```python
from build123d import *

# Parameters (mm, degrees)
F0_R     = 12.7
F2_DEPTH = 362.63707
F3_D     = 19.05


with BuildPart() as f2:
    # F0 (on Right) → F2 (new body)
    with BuildSketch(Plane.YZ):
        Circle(F0_R)
    extrude(amount=F2_DEPTH)

    # F3 (through all)
    with Locations(Plane(origin=(0, 0, 0), x_dir=(0, 1, 0), z_dir=(-1, 0, 0))):
        with Locations((0, 0)):
            Hole(F3_D / 2)

    # F4: F2 across plane


with BuildPart() as f2_1:
    add(f2.part)
    add(f2.part.mirror(Plane.YZ))


solid = f2_1.part
```
Design review of the part built by this model. Coordinates are the model's own, in mm. Round coordinates to 2 decimals unless told otherwise and drop trailing zeros. Order: outer loops, then holes, each group sorted by start corner. A loop starts at its lowest first (then second) coordinate and runs counter-clockwise, first axis right, second up. Notation, with made-up numbers: M 33,-29 L 60,-29 A6 cw 60,-23 Z; hole C 39.5,30 d9. An arc over 180 degrees is marked long. Put each result on its own line as item: value.
Q1. Draft analysis for pull direction Y (two halves, no side actions). For faces 1 (the face through (5.08, -2.75, -12.4)), 2 (the face through (-5.077, 7.559, 5.796)), 3 (the face through (362.637, 5, 9)), state which applies: released by +Y, released by -Y, zero draft, split by the parting line, or undercut.
Reported:
face 1: split by the parting line
face 2: undercut
face 3: zero draft
Q2. To check wall thickness, follow line 1 (Z direction, x = -6, y = 0) (3 decimals); line 2 (Z direction, x = -159, y = 1.25); line 3 (Y direction, x = -307, z = -0.75). State the ranges of each line that lie inside material, in increasing order.
Reported:
line 1: -12.7 to -9.525, 9.525 to 12.7
line 2: -12.64 to -9.44, 9.44 to 12.64
line 3: -12.68 to -9.5, 9.5 to 12.68
Q3. Consider section A-A (y = 0). State the section outline as (x, z) points (3 decimals).
Reported:
outline: M -362.637,-12.7 L 362.637,-12.7 L 362.637,-9.525 L -362.637,-9.525 Z; M -362.637,9.525 L 362.637,9.525 L 362.637,12.7 L -362.637,12.7 Z
Q4. Consider section C-C (x = -95.5). State the section outline as (y, z) points (3 decimals).
Reported:
outline: C 0,0 d25.4; hole C 0,0 d19.05
Q5. Insertion check: pin 1 Ø1.5 at (x, z) = (-223.5, 2) entering from +Y; pin 2 Ø6 at (x, y) = (-236, -9) entering from +Z; pin 3 Ø3 at (x, z) = (-67, -7) entering from +Y. Each pin has a flat end and moves straight along its axis. Give the tip position at first contact, or say it passes through.
Reported:
pin 1: y = 12.64
pin 2: z = 11.19
pin 3: y = 11.45
